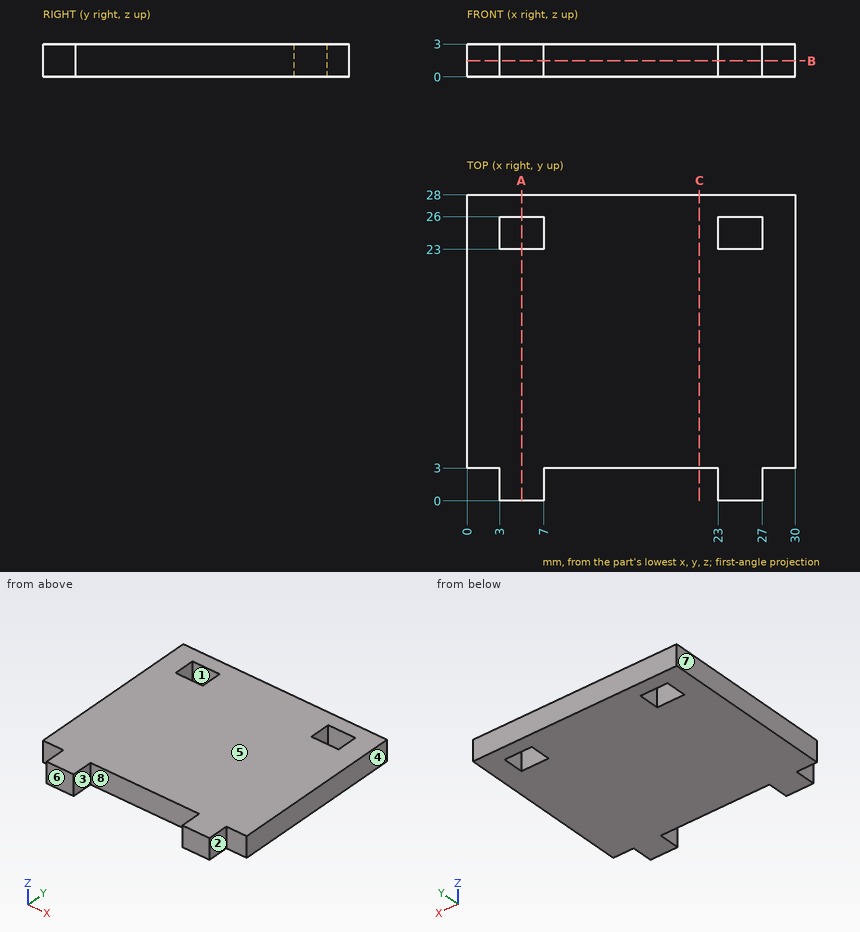
Answer from the drawing. Dimensions are ordinates in mm from the lowest x, y and z of the part. A direction names the side the tool comes from. Round coordinates to 2 decimals unless told otherwise and drop trailing zeros. Write each loop counter-clockwise with the first axis right and the second up, starting at its lowest first coordinate (ties: lowest second). Pieces come first, ordered by that corner, then holes. Notation, with made-up numbers: (38.5, 1) - (43.5, 1) arc R17 cw to (43.5, 7) - close; hole circle Ø7 at (-13, -18). An arc over 180 degrees is marked (long way). Use a Markdown table: item, result.
(1) The mould has two halves that part along X. Classify the marked faces 6, 7 and 8: released by +X, released by -X, zero draft, split by the parting line, or undercut.
Reported:
| item | result |
|---|---|
| face 6 | zero draft |
| face 7 | released by -X |
| face 8 | undercut |
(2) The part is cut by section A-A (x = 5). Write down the section's boundary in (y, z).
Reported:
| item | result |
|---|---|
| outline | (0, 0) - (23, 0) - (23, 3) - (0, 3) - close; (26, 0) - (28, 0) - (28, 3) - (26, 3) - close |
(3) Which of the six approach directions +Z, -Z, +X, -X, +Y, -Y give full straight-line access (tool end or side, diameter ignored) to the marked faces 1, 2, 3, 4 and 5?
Reported:
| item | result |
|---|---|
| face 1 | +Z, -Z |
| face 2 | +Z, -Z, +X, -Y |
| face 3 | +Z, -Z, -Y |
| face 4 | +Z, -Z, +X, +Y, -Y |
| face 5 | +Z, +X, -X, +Y, -Y |
(4) The part is cut by section C-C (x = 21.25). Write down the section's boundary in (y, z), then the cut area to 3 significant figures.
Reported:
| item | result |
|---|---|
| outline | (3, 0) - (28, 0) - (28, 3) - (3, 3) - close |
| area | 75.0 mm2 |
(5) The part is cut by section B-B (z = 1.45). Write down the section's boundary in (x, y), then the cut area to 3 significant figures.
Reported:
| item | result |
|---|---|
| outline | (0, 3) - (3, 3) - (3, 0) - (7, 0) - (7, 3) - (23, 3) - (23, 0) - (27, 0) - (27, 3) - (30, 3) - (30, 28) - (0, 28) - close; hole (3, 23) - (7, 23) - (7, 26) - (3, 26) - close; hole (23, 23) - (27, 23) - (27, 26) - (23, 26) - close |
| area | 750 mm2 |
(6) Each of these flat-tipped pins is pushed along its axis until it touches: pin 1 Ø0.9 at (y, z) = (1.5, 1) entering from -X; pin 2 Ø0.9 at (y, z) = (1, 1.5) entering from +X. Where does it stop, or does it pass through?
Reported:
| item | result |
|---|---|
| pin 1 | x = 3 |
| pin 2 | x = 27 |
(7) Straight lines are drawn through the part: line 1 along X through (y, z) = (24.5, 1.95); line 2 along Y through (x, z) = (4, 0.65); line 3 along Y through (x, z) = (28.25, 1). For each, find the intervals that lie inside material, in ascending order. Write a range as [from, to].
Reported:
| item | result |
|---|---|
| line 1 | [0, 3], [7, 23], [27, 30] |
| line 2 | [0, 23], [26, 28] |
| line 3 | [3, 28] |
